The model under review builds one solid part; all positions refer to its coordinate system, in mm. Face numbers are marked on the shaded views. A direction names the side the tool comes from. Round coordinates to 2 decimals unless told otherwise and drop trailing zeros. Order: outer loops, then holes, each group sorted by start corner. A loop starts at its lowest first (then second) coordinate and runs counter-clockwise, first axis right, second up.
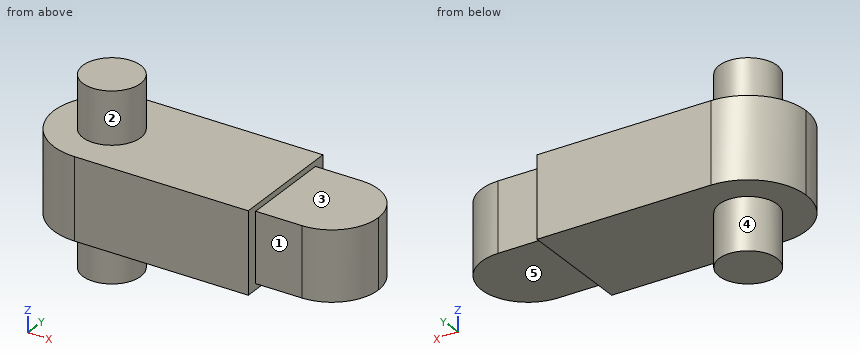
Autodesk Inventor part; units mm, degrees
ref_plane "YZ Plane" through (0, 0, 0) normal (1, 0, 0) x (0, 1, 0)
ref_plane "XZ Plane" through (0, 0, 0) normal (0, 1, 0) x (-1, 0, 0)
sketch "스케치1" plane through (0, 0, 0) normal (0, 0, 1) x (1, 0, 0)
  line L0 (-10, 5) -> (10, 5)
  line L1 (10, 5) -> (10, -5)
  line L2 (10, -5) -> (-10, -5)
  line L3 (-10, -5) -> (-10, 5)
  line L4 (-10, 5) -> (10, -5) construction
  line L5 (10, 5) -> (-10, -5) construction
  line L6 (10, 4) -> (18, 4)
  line L7 (18, 4) -> (18, -4)
  line L8 (18, -4) -> (10, -4)
  line L9 (10, -4) -> (10, 4)
  circle A0 centre (-5, 0) radius 2.5
  point P0 (0, 0)
  point P1 (0, 0)
  point P2 (18, 0)
  dimension "d0" = 20
  dimension "d1" = 10
  dimension "d2" = 8
  dimension "d3" = 8
  dimension "d4" = 5
  dimension "d5" = 15
  dimension "d6" = 5
extrude "돌출1" add sketch "스케치1" along normal mid plane 16 contours A0
extrude "돌출2" add sketch "스케치1" along normal mid plane 7 contours L0 L1 L2 L3
extrude "돌출3" add sketch "스케치1" along normal mid plane 6 contours L6 L7 L8 L1
fillet "모깎기1" radius 4 2 edges at (18, 4, 0) (18, -4, 0)
fillet "모깎기2" radius 5 2 edges at (-10, 5, 0) (-10, -5, 0)
properties part number "03-2"
(1) To check wall thickness, follow L1, parallel to Z at x = -3.5, y = 3; L2, parallel to Z at x = 10.5, y = 3; L3, parallel to Y at x = -7.25, z = 0.25. State the ranges of each line that lie inside material, in increasing order.
(2) We need section D-D (y = -2). Give the boundary of the cut face in (x, z), and give its area (3 significant figures).
(3) We need section B-B (y = 1.5). Give the boundary of the cut face in (x, z), and give its area (3 significant figures).
(4) Tool access review of the marked faces 1, 2, 3, 4 and 5: name each direction out of +Z, -Z, +X, -X, +Y, -Y from which nothing blocks a thin tool from reaching the whole face with its end or side.
(5) We need section C-C (x = -5.5). Give the boundary of the cut face in (y, z), and give its area (3 significant figures).
(6) Clearance check with flat-ended pins moving along their axes: P1, Ø1.2, axis at x = 12.5, z = -1, coming from the +Y side; P2, Ø2, axis at y = 0.5, z = -6, coming from the +X side; P3, Ø3, axis at y = -2, z = -1.5, coming from the -X side (3 decimals). State where each tip first meets the part, or that it passes through.
Verdict:
1. L1: z = -3.5 to 3.5
1. L2: z = -3 to 3
1. L3: y = -4.47 to 4.47
2. outline: (-9.58, -3.5) - (-6.5, -3.5) - (-6.5, -8) - (-3.5, -8) - (-3.5, -3.5) - (10, -3.5) - (10, -3) - (17.46, -3) - (17.46, 3) - (10, 3) - (10, 3.5) - (-3.5, 3.5) - (-3.5, 8) - (-6.5, 8) - (-6.5, 3.5) - (-9.58, 3.5) - close
2. area: 209 mm2
3. outline: (-9.77, -3.5) - (-7, -3.5) - (-7, -8) - (-3, -8) - (-3, -3.5) - (10, -3.5) - (10, -3) - (17.71, -3) - (17.71, 3) - (10, 3) - (10, 3.5) - (-3, 3.5) - (-3, 8) - (-7, 8) - (-7, 3.5) - (-9.77, 3.5) - close
3. area: 221 mm2
4. face 1: +Z, -Z, +X, -Y
4. face 2: +Z
4. face 3: +Z, +X, +Y, -Y
4. face 4: -Z
4. face 5: -Z, +X, +Y, -Y
5. outline: (-4.97, -3.5) - (-2.45, -3.5) - (-2.45, -8) - (2.45, -8) - (2.45, -3.5) - (4.97, -3.5) - (4.97, 3.5) - (2.45, 3.5) - (2.45, 8) - (-2.45, 8) - (-2.45, 3.5) - (-4.97, 3.5) - close
5. area: 114 mm2
6. P1: stops at y = 4
6. P2: stops at x = -2.5
6. P3: stops at x = -9.975
